Could you check a few things on this drawing? It's one solid part, dimensions in mm from its lowest x, y, z. Round coordinates to 2 decimals unless told otherwise and drop trailing zeros. Order: outer loops, then holes, each group sorted by start corner. A loop starts at its lowest first (then second) coordinate and runs counter-clockwise, first axis right, second up. Notation, with made-up numbers: (-16.75, 18.5) - (2.25, 18.5) arc R11 cw to (2.25, 31.5) - close; hole circle Ø8 at (76.25, 10). An arc over 180 degrees is marked (long way). Use one line per item in the form item = value.
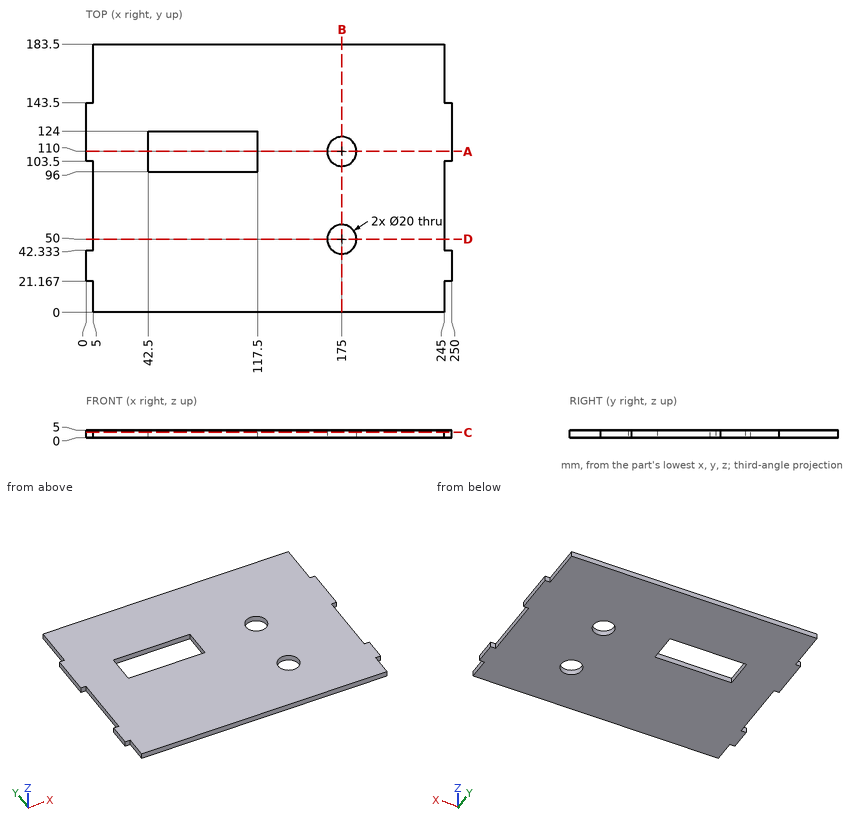
Item 1: Will these pins go through, and if not, where does the flat tip stop? P1, Ø1.5, axis at x = 3.5, z = 1.5, coming from the -Y side; P2, Ø1.5, axis at y = 60, z = 3, coming from the +X side; P3, Ø1.5, axis at x = 246.5, z = 3, coming from the +Y side.
Found:
P1 = 21.17
P2 = 245
P3 = 143.5
Item 2: I need wall thicknesses on L1, parallel to Y at x = 175, z = 3.6; L2, parallel to X at y = 109.5, z = 2.95; L3, parallel to X at y = 121, z = 0.2. Which ranges of each line are inside material? Lowest first, please.
Found:
L1 = 0 to 40, 60 to 100, 120 to 183.5
L2 = 0 to 42.5, 117.5 to 165.01, 184.99 to 250
L3 = 0 to 42.5, 117.5 to 250
Item 3: Imagine slicing it at B-B on x = 175. Please give me the cut outline in (y, z).
Found:
outline = (0, 0) - (40, 0) - (40, 5) - (0, 5) - close; (60, 0) - (100, 0) - (100, 5) - (60, 5) - close; (120, 0) - (183.5, 0) - (183.5, 5) - (120, 5) - close
Item 4: Imagine slicing it at D-D on y = 50. Please give me the cut outline in (x, z).
Found:
outline = (5, 0) - (165, 0) - (165, 5) - (5, 5) - close; (185, 0) - (245, 0) - (245, 5) - (185, 5) - close
Item 5: Imagine slicing it at C-C on z = 3.7. Please give me the cut outline in (x, y), plus the area to 3 significant figures.
Found:
outline = (0, 21.17) - (5, 21.17) - (5, 0) - (245, 0) - (245, 21.17) - (250, 21.17) - (250, 42.33) - (245, 42.33) - (245, 103.5) - (250, 103.5) - (250, 143.5) - (245, 143.5) - (245, 183.5) - (5, 183.5) - (5, 143.5) - (0, 143.5) - (0, 103.5) - (5, 103.5) - (5, 42.33) - (0, 42.33) - close; hole (42.5, 96) - (117.5, 96) - (117.5, 124) - (42.5, 124) - close; hole circle Ø20 at (175, 50); hole circle Ø20 at (175, 110)
area = 41,900 mm2
Item 6: Imagine slicing it at A-A on y = 110. Please give me the cut outline in (x, z), plus the area to 3 significant figures.
Found:
outline = (0, 0) - (42.5, 0) - (42.5, 5) - (0, 5) - close; (117.5, 0) - (165, 0) - (165, 5) - (117.5, 5) - close; (185, 0) - (250, 0) - (250, 5) - (185, 5) - close
area = 775 mm2
